```python
from build123d import *

# Parameters (mm, degrees)
SKETCH1_R           = 35
SKETCH1_R_2         = 25
BOSS_EXTRUDE1_DEPTH = 90
BOSS_EXTRUDE2_START = -20
SKETCH1_3_R         = 15
SKETCH1_3_R_2       = 7.5
BOSS_EXTRUDE2_DEPTH = 15
BOSS_EXTRUDE3_START = -65
SKETCH1_4_R         = 7.5
BOSS_EXTRUDE3_DEPTH = 15


with BuildPart() as part:
    # Sketch1 → Boss-Extrude1 (new body)
    with BuildSketch(Plane(origin=(0, 0, 0), x_dir=(1, 0, 0), z_dir=(0, 1, 0))):
        with Locations(Location((0, 0, 0), (0, 0, 270))):
            Circle(SKETCH1_R)
        with Locations(Location((0, 0, 0), (0, 0, 270))):
            Circle(SKETCH1_R_2, mode=Mode.SUBTRACT)
    extrude(amount=-BOSS_EXTRUDE1_DEPTH)

    # Sketch1_3 → Boss-Extrude2 (add)
    # profile 1 of 3: a face of its own
    with BuildSketch(Plane(origin=(0, 0, 0), x_dir=(1, 0, 0), z_dir=(0, 1, 0)).offset(BOSS_EXTRUDE2_START)):
        with Locations((80, 0)):
            Circle(SKETCH1_3_R)
        with Locations(Location((80, 0, 0), (0, 0, 270))):
            Circle(SKETCH1_3_R_2, mode=Mode.SUBTRACT)
    # profile 2 of 3: a face of its own
    with BuildSketch(Plane(origin=(0, 0, 0), x_dir=(1, 0, 0), z_dir=(0, 1, 0)).offset(BOSS_EXTRUDE2_START)):
        with BuildLine():
            Line((25, -24.494897428), (25, -29.692872321))
            Line((25, -29.692872321), (83.75, -14.523687548))
            ThreePointArc((83.75, -14.523687548), (65, 0), (83.75, 14.523687548))
            Line((83.75, 14.523687548), (8.75, 33.888604279))
            ThreePointArc((8.75, 33.888604279), (27.669929526, 21.433035249), (35, 0))
            ThreePointArc((35, 0), (32.403703492, -13.228756555), (25, -24.494897428))
        make_face()
    # profile 3 of 3: a face of its own
    with BuildSketch(Plane(origin=(0, 0, 0), x_dir=(1, 0, 0), z_dir=(0, 1, 0)).offset(BOSS_EXTRUDE2_START)):
        with BuildLine():
            Line((8.75, -33.888604279), (25, -29.692872321))
            Line((25, -29.692872321), (25, -24.494897428))
            ThreePointArc((25, -24.494897428), (17.516451042, -30.301385165), (8.75, -33.888604279))
        make_face()
    extrude(amount=-BOSS_EXTRUDE2_DEPTH)

    # Sketch1_4 → Boss-Extrude3 (add)
    with BuildSketch(Plane(origin=(0, 0, 0), x_dir=(1, 0, 0), z_dir=(0, 1, 0)).offset(BOSS_EXTRUDE3_START)):
        with BuildLine():
            ThreePointArc((-35, -60), (-5, -90), (25, -60))
            Line((25, -60), (25, -29.692872321))
            Line((25, -29.692872321), (8.75, -33.888604279))
            ThreePointArc((8.75, -33.888604279), (-21.433035249, -27.669929526), (-35, 0))
            Line((-35, 0), (-35, -60))
        make_face()
        with Locations(Location((-5, -60, 0), (0, 0, 270))):
            Circle(SKETCH1_4_R, mode=Mode.SUBTRACT)
    extrude(amount=-BOSS_EXTRUDE3_DEPTH)


solid = part.part
```
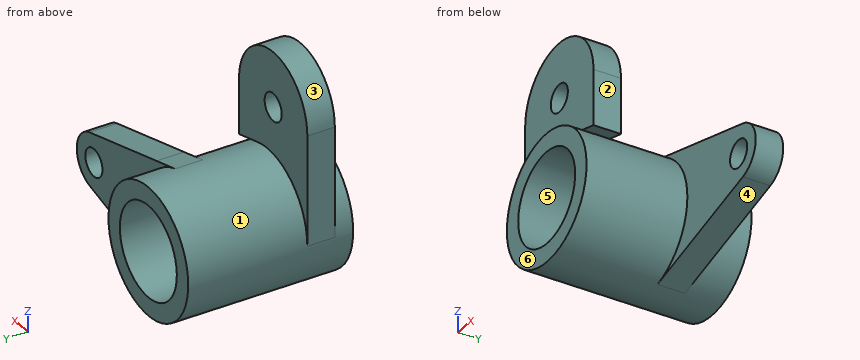
Model file for the job. Use its own axes, mm. Face numbers are marked on the shaded views. A direction names the side the tool comes from. Coordinates: 2 decimals unless noted, no trailing zeros. Loops run counter-clockwise (first coordinate to the right, second up) from the corner with the lowest first, then second, coordinate; pieces in that order, holes last. Notation, with made-up numbers: (27.5, 38.25) - (32.5, 38.25) arc R25 cw to (32.5, 76.25) - close; hole circle Ø4 at (42.25, 9.25). An arc over 180 degrees is marked (long way). Answer as a JSON object with one key per item and string values. Group by question number.
(1) Cut at C-C (y = -27.5). Give the cut face in (x, z).
(2) Cut at D-D (z = 62.5). Give the cut face in (x, y).
(3) Cut at B-B (z = 5). Give the cut face in (x, y), then the cut area to 3 significant figures.
(4) Flat gauge pins, fed straight in: pin 1 (19.5 mm diameter, centred on x = 80, z = 0, fed in from -Y); pin 2 (5 mm diameter, centred on x = 40, z = 7, fed in from +Y); pin 3 (4 mm diameter, centred on x = -15, y = -70, fed in from -Z). Where does each tip first touch, or does it go through?
(5) Tool access for the marked faces 1, 2 and 3: list every direction of +Z, -Z, +X, -X, +Y, -Y with a clear straight run to the whole face (end or side of a thin tool).
(6) Two-plate mould, pull along X, no slides. Class the marked faces 4, 5 and 6: released by +X, released by -X, zero draft, split by the parting line, or undercut.
(7) Cut at A-A (x = 78). Give the cut face in (y, z), then the cut area to 3 significant figures.
(8) Probe line 1 along X through (y, z) = (-24, 0); line 2 along X through (y, z) = (-70.5, 60); line 3 along Y through (x, z) = (3.5, 78). List the from-to ranges inside material, lowest first.
Geometry says:
{
 "1": {"outline": "(8.75, -33.89) - (83.75, -14.52) arc R15 ccw to (83.75, 14.52) - (8.75, 33.89) arc R35 ccw (long way) to start; hole circle Ø50 at (0, 0); hole circle Ø15 at (80, 0)"},
 "2": {"outline": "(-34.9, -80) - (-12.07, -80) - (-12.07, -65) - (-34.9, -65) - close; (2.07, -80) - (24.9, -80) - (24.9, -65) - (2.07, -65) - close"},
 "3": {"outline": "(-35, -80) - (-34.64, -80) - (-34.64, -90) - (-24.49, -90) - (-24.49, 0) - (-34.64, 0) - (-34.64, -65) - (-35, -65) - close; (24.49, -90) - (34.64, -90) - (34.64, -35) - (74.41, -35) - (74.41, -20) - (34.64, -20) - (34.64, 0) - (24.49, 0) - close; (85.59, -35) - (94.14, -35) - (94.14, -20) - (85.59, -20) - close", "area": "2,560 mm^2"},
 "4": {"pin 1": "stops at y = -35", "pin 2": "stops at y = -20", "pin 3": "stops at z = -32.5"},
 "5": {"face 1": "none", "face 2": "+Z, +X, +Y, -Y", "face 3": "+Z, +Y, -Y"},
 "6": {"face 4": "released by +X", "face 5": "undercut", "face 6": "zero draft"},
 "7": {"outline": "(-35, -16.01) - (-20, -16.01) - (-20, -7.23) - (-35, -7.23) - close; (-35, 7.23) - (-20, 7.23) - (-20, 16.01) - (-35, 16.01) - close", "area": "263 mm^2"},
 "8": {"line 1": "x = -35 to -25, 25 to 72.5, 87.5 to 95", "line 2": "x = -35 to -12.5, 2.5 to 25", "line 3": "y = -80 to -65"}
}
